```python
from build123d import *

# Parameters (mm, degrees)
SKETCH2_R          = 4.7625
BODY_EXTRUDE_DEPTH = 4.7625
BODY_FILLET_A_R    = 1.016
BODY_FILLET_B_R    = 1.016
CHAMFER2_SIZE      = 1.016
ID_CHAMFER_SIZE    = 0.381
SKETCH3_R          = 2.5796875
HOLE_CUT_DEPTH     = 24.65886697


with BuildPart() as part:
    # Sketch2 → Body Extrude (new, symmetric)
    with BuildSketch(Plane.XY):
        with BuildLine():
            Line((-18.25625, 0), (-18.25625, 4.7752))
            Line((-18.25625, 4.7752), (-9.525, 4.7752))
            Line((-9.525, 4.7752), (-9.525, 9.525))
            ThreePointArc((-9.525, 9.525), (0, 19.05), (9.525, 9.525))
            Line((9.525, 9.525), (9.525, 4.7752))
            Line((9.525, 4.7752), (18.25625, 4.7752))
            Line((18.25625, 4.7752), (18.25625, 0))
            Line((18.25625, 0), (-18.25625, 0))
        make_face()
        with Locations(Location((0, 9.525, 0), (0, 0, 180))):
            Circle(SKETCH2_R, mode=Mode.SUBTRACT)
    extrude(amount=BODY_EXTRUDE_DEPTH, both=True)

    # Body Fillet A
    body_fillet_a_edges = [part.edges().sort_by_distance(p)[0] for p in [
        (9.525, 7.1501, 4.7625),
        (0, 19.05, 4.7625),
        (-9.525, 7.1501, 4.7625),
        (-9.525, 7.1501, -4.7625),
        (0, 19.05, -4.7625),
        (9.525, 7.1501, -4.7625),
    ]]
    fillet(body_fillet_a_edges, radius=BODY_FILLET_A_R)

    # Body Fillet B
    # the kernel refuses this fillet: 1.016 mm, written as the material it adds along each edge
    with BuildSketch(Plane(origin=(-9.525, 4.7752, 3.7465), x_dir=(0, 1, 0), z_dir=(0, 0, -1))) as body_fillet_b_piece_1:
        with BuildLine():
            CenterArc((BODY_FILLET_B_R, -BODY_FILLET_B_R), BODY_FILLET_B_R, 90, 90)
            Line((0, -BODY_FILLET_B_R), (0, 0))
            Line((0, 0), (BODY_FILLET_B_R, 0))
        make_face()
    extrude(amount=7.493)
    with BuildSketch(Plane(origin=(9.525, 4.7752, 3.7465), x_dir=(0, 1, 0), z_dir=(0, 0, -1))) as body_fillet_b_piece_2:
        with BuildLine():
            CenterArc((BODY_FILLET_B_R, BODY_FILLET_B_R), BODY_FILLET_B_R, 180, 90)
            Line((0, BODY_FILLET_B_R), (0, 0))
            Line((0, 0), (BODY_FILLET_B_R, 0))
        make_face()
    extrude(amount=7.493)
    with BuildSketch(Plane(origin=(-8.509, 4.7752, -3.7465), x_dir=(-1, 0, 0), z_dir=(0, 0, 1))) as body_fillet_b_piece_3_section:
        with BuildLine():
            CenterArc((1.016 + BODY_FILLET_B_R, -BODY_FILLET_B_R), BODY_FILLET_B_R, 90, 90)
            Line((1.016 + BODY_FILLET_B_R, 0), (1.016, 0))
            Line((1.016, 0), (1.016, -BODY_FILLET_B_R))
        make_face()
    body_fillet_b_piece_3 = revolve(axis=Axis((-8.509, 4.7752, -3.7465), (0, -1, 0)), revolution_arc=233.296989237, mode=Mode.PRIVATE)
    body_fillet_b_piece_3 = split(body_fillet_b_piece_3, bisect_by=Plane(origin=(-9.270938019, 5.091814151, -4.7625), z_dir=(0, 0, 1)), keep=Keep.TOP, mode=Mode.PRIVATE)
    add(body_fillet_b_piece_3)
    with BuildSketch(Plane(origin=(8.509, 4.7752, 3.7465), x_dir=(-0.5976672776328273, 0, -0.8017442392976483), z_dir=(0.8017442392976483, 0, -0.5976672776328273))) as body_fillet_b_piece_4_section:
        with BuildLine():
            CenterArc((1.016 + BODY_FILLET_B_R, BODY_FILLET_B_R), BODY_FILLET_B_R, 180, 90)
            Line((1.016, BODY_FILLET_B_R), (1.016, 0))
            Line((1.016, 0), (1.016 + BODY_FILLET_B_R, 0))
        make_face()
    body_fillet_b_piece_4 = revolve(axis=Axis((8.509, 4.7752, 3.7465), (0, 1, 0)), revolution_arc=233.296989237, mode=Mode.PRIVATE)
    body_fillet_b_piece_4 = split(body_fillet_b_piece_4, bisect_by=Plane(origin=(9.270937806, 5.091814769, 4.7625), z_dir=(0, 0, -1)), keep=Keep.TOP, mode=Mode.PRIVATE)
    add(body_fillet_b_piece_4)
    with BuildSketch(Plane(origin=(8.509, 4.7752, -3.7465), x_dir=(1, 0, 0), z_dir=(0, 0, 1))) as body_fillet_b_piece_5_section:
        with BuildLine():
            CenterArc((1.016 + BODY_FILLET_B_R, BODY_FILLET_B_R), BODY_FILLET_B_R, 180, 90)
            Line((1.016 + BODY_FILLET_B_R, 0), (1.016, 0))
            Line((1.016, 0), (1.016, BODY_FILLET_B_R))
        make_face()
    body_fillet_b_piece_5 = revolve(axis=Axis((8.509, 4.7752, -3.7465), (0, 1, 0)), revolution_arc=233.296989237, mode=Mode.PRIVATE)
    body_fillet_b_piece_5 = split(body_fillet_b_piece_5, bisect_by=Plane(origin=(9.270937903, 5.091814444, -4.7625), z_dir=(0, 0, 1)), keep=Keep.TOP, mode=Mode.PRIVATE)
    add(body_fillet_b_piece_5)
    with BuildSketch(Plane(origin=(-8.509, 4.7752, 3.7465), x_dir=(0.5976672776328271, 0, -0.8017442392976484), z_dir=(-0.8017442392976484, 0, -0.5976672776328271))) as body_fillet_b_piece_6_section:
        with BuildLine():
            CenterArc((1.016 + BODY_FILLET_B_R, -BODY_FILLET_B_R), BODY_FILLET_B_R, 90, 90)
            Line((1.016 + BODY_FILLET_B_R, 0), (1.016, 0))
            Line((1.016, 0), (1.016, -BODY_FILLET_B_R))
        make_face()
    body_fillet_b_piece_6 = revolve(axis=Axis((-8.509, 4.7752, 3.7465), (0, -1, 0)), revolution_arc=233.296989237, mode=Mode.PRIVATE)
    body_fillet_b_piece_6 = split(body_fillet_b_piece_6, bisect_by=Plane(origin=(-9.270937967, 5.09181436, 4.7625), z_dir=(0, 0, -1)), keep=Keep.TOP, mode=Mode.PRIVATE)
    add(body_fillet_b_piece_6)

    # Chamfer2
    chamfer2_edges = [part.edges().sort_by_distance(p)[0] for p in [
        (18.25625, 2.3876, -4.7625),
        (-18.25625, 2.3876, 4.7625),
        (18.25625, 2.3876, 4.7625),
        (-18.25625, 2.3876, -4.7625),
    ]]
    chamfer(chamfer2_edges, length=CHAMFER2_SIZE)

    # ID Chamfer
    id_chamfer_edges = [part.edges().sort_by_distance(p)[0] for p in [
        (4.7625, 9.525, -4.7625),
        (4.7625, 9.525, 4.7625),
    ]]
    chamfer(id_chamfer_edges, length=ID_CHAMFER_SIZE)

    # Sketch3 → Hole Cut (cut, through all)
    with BuildSketch(Plane(origin=(0, 4.7752, 0), x_dir=(1, 0, 0), z_dir=(0, 1, 0))):
        with Locations(Location((-14.2875, 0, 0), (0, 0, 180))):
            Circle(SKETCH3_R)
        with Locations((14.2875, 0)):
            Circle(SKETCH3_R)
    extrude(amount=-HOLE_CUT_DEPTH, mode=Mode.SUBTRACT)


solid = part.part
```
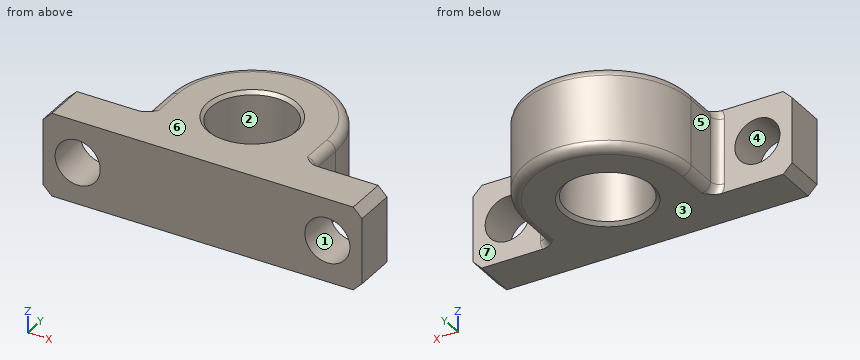
Design review of the part built by this model. Coordinates are the model's own, in mm. Face numbers are marked on the shaded views. A direction names the side the tool comes from. Give positions to 0.01 mm unless a question says otherwise; leave off trailing zeros. Loops run counter-clockwise (first coordinate to the right, second up) from the corner with the lowest first, then second, coordinate; pieces in that order, holes last. Notation, with made-up numbers: (86.5, 73) -> (141.5, 73) arc R29 cw to (141.5, 99) -> close; hole circle Ø1 at (-9.75, 43.5). An arc over 180 degrees is marked (long way). Write each question's results on one line, items separated by ' | '.
Q1. Take a section at A-A, the plane z = 0. Give the number of separate pieces and of enclosed holes in the cut face, plus the area to 3 significant figures.
Reply:
separate pieces: 3 | enclosed holes: 1 | area: 287 mm²
Q2. Wall thickness on L1, parallel to Y at x = 0, z = 1.75; L2, parallel to X at y = 3.25, z = 1.75; L3, parallel to Y at x = -16, z = -2: over which ranges is each line inside the solid? List them lowest first.
Reply:
L1: y = 0 to 4.76, 14.29 to 19.05 | L2: x = -18.26 to -16.18, -12.39 to 12.39, 16.18 to 18.26 | L3: y = 0 to 4.78
Q3. For pin 1 Ø4 at (x, z) = (14.29, 0) entering from -Y; pin 2 Ø4 at (x, z) = (13, 2) entering from +Y; pin 3 Ø2 at (x, z) = (5, -3.5) entering from +Y; pin 4 Ø3 at (y, z) = (8.5, -1) entering from +X (3 decimals), all flat-tipped, find the tip position at first contact; note any pin that passes through.
Reply:
pin 1: passes through | pin 2: stops at y = 4.78 | pin 3: stops at y = 18.17 | pin 4: stops at x = 9.525
Q4. Take a section at C-C, the plane y = 2. Write out the cut boundary in (x, z).
Reply:
outline: (-18.26, -3.75) -> (-17.24, -4.76) -> (17.24, -4.76) -> (18.26, -3.75) -> (18.26, 3.75) -> (17.24, 4.76) -> (-17.24, 4.76) -> (-18.26, 3.75) -> close; hole circle Ø5.16 at (-14.29, 0); hole circle Ø5.16 at (14.29, 0)
Q5. Machinability: for the marked faces 5, 6 and 7, which of the approach directions +Z, -Z, +X, -X, +Y, -Y give a long, thin tool a straight path to every point of the face, cutting with its end or side? Answer none if there is none.
Reply:
face 5: +Z, -Z, -X, +Y | face 6: +Z, +X, -X, +Y, -Y | face 7: +Z, -Z, +X, +Y
Q6. The part is to be moulded in two halves that separate along Z. For the marked faces 1, 2, 3 and 4, say which applies: +Z half, -Z half, draft (parallel to the pull), parting line (faces both ways), or undercut.
Reply:
face 1: undercut | face 2: draft | face 3: -Z half | face 4: undercut
Q7. Take a section at B-B, the plane x = 0. Write out the cut boundary in (y, z).
Reply:
outline: (0, -4.76) -> (4.38, -4.76) -> (4.76, -4.38) -> (4.76, 4.38) -> (4.38, 4.76) -> (0, 4.76) -> close; (14.29, -4.38) -> (14.67, -4.76) -> (18.03, -4.76) arc R1.02 ccw to (19.05, -3.75) -> (19.05, 3.75) arc R1.02 ccw to (18.03, 4.76) -> (14.67, 4.76) -> (14.29, 4.38) -> close
